from build123d import *

# Parameters (mm, degrees)
PAD_DEPTH       = 100
POCKET_DEPTH    = 35
SKETCH002_W     = 180
SKETCH002_H     = 35
POCKET001_DEPTH = 77
POCKET002_DEPTH = 27


with BuildPart() as part:
    # Sketch001 → Pad (new body)
    with BuildSketch(Plane.XY):
        with BuildLine():
            ThreePointArc((99, 7.5), (80.254858, 52.75481), (35.000067, 71.5))
            Line((35.000067, 71.5), (-35, 71.5))
            ThreePointArc((-35, 71.5), (-80.254834, 52.754834), (-99, 7.5))
            Line((-99, 7.5), (-99, -7.5))
            ThreePointArc((-99, -7.5), (-80.254834, -52.754834), (-35, -71.5))
            Line((-35, -71.5), (35.000001, -71.5))
            ThreePointArc((35.000001, -71.5), (80.254834, -52.754834), (99, -7.5))
            Line((99, 7.5), (99, -7.5))
        make_face()
    extrude(amount=PAD_DEPTH)

    # Sketch → Pocket (cut)
    with BuildSketch(Plane.XY.offset(30)):
        with BuildLine():
            ThreePointArc((89, 7.5), (73.183766, 45.683767), (34.999999, 61.5))
            Line((34.999999, 61.5), (-35, 61.5))
            ThreePointArc((-35, 61.5), (-73.183766, 45.683766), (-89, 7.5))
            Line((-89, 7.5), (-89, -7.5))
            ThreePointArc((-89, -7.5), (-73.183766, -45.683766), (-35, -61.5))
            Line((-35, -61.5), (35, -61.5))
            ThreePointArc((35, -61.5), (73.183766, -45.683766), (89, -7.5))
            Line((89, 7.5), (89, -7.5))
        make_face()
    extrude(amount=POCKET_DEPTH, mode=Mode.SUBTRACT)

    # Sketch002 → Pocket001 (cut)
    with BuildSketch(Plane.XZ.offset(80)):
        with Locations((0, 47.5)):
            Rectangle(SKETCH002_W, SKETCH002_H)
    extrude(amount=-POCKET001_DEPTH, mode=Mode.SUBTRACT)

    # Sketch003 → Pocket002 (cut)
    with BuildSketch(Plane.XY):
        with BuildLine():
            ThreePointArc((96, 7.5), (78.133514, 50.633513), (35.000001, 68.5))
            Line((35.000001, 68.5), (-35, 68.5))
            ThreePointArc((-35, 68.5), (-78.133514, 50.633514), (-96, 7.5))
            Line((-96, 7.5), (-96, -7.5))
            ThreePointArc((-96, -7.5), (-78.133514, -50.633514), (-35, -68.5))
            Line((-35, -68.5), (34.999897, -68.5))
            ThreePointArc((34.999897, -68.5), (78.133477, -50.63355), (96, -7.5))
            Line((96, 7.5), (96, -7.5))
        make_face()
    extrude(amount=POCKET002_DEPTH, mode=Mode.SUBTRACT)


solid = part.part
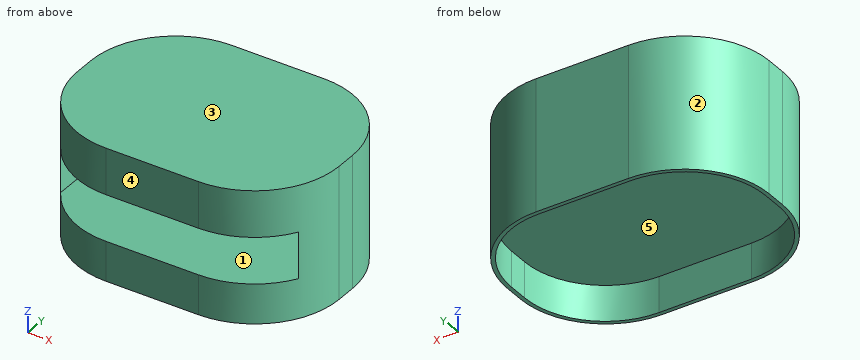
Verification items for the finished model (mm, model axes). Face numbers are marked on the shaded views. A direction names the side the tool comes from. Give positions to 0.01 mm unless a question says otherwise; leave off trailing zeros. Write each loop counter-clockwise with the first axis right and the second up, starting at its lowest first coordinate (ties: lowest second). Pieces come first, ordered by that corner, then holes.
(1) Cross-section at C-C (y = 52). Enter the section's corners in (x, z), plus the area to 3 significant figures.
(2) Access from +Z, -Z, +X, -X, +Y, -Y to the whole of each face (thin tool, end or side, straight path). Record for the marked faces 4 and 5.
(3) Material ranges on line 1 (Z direction, x = 33, y = 61); line 2 (Y direction, x = 32, z = 26); line 3 (Y direction, x = 22, z = 43), recorded low to high.
(4) Gauge pin test, flat ends, axial feed: pin 1 (2 mm diameter, centred on x = -72, z = 63.5, fed in from +Y) (3 decimals); pin 2 (2 mm diameter, centred on y = 31, z = 23, fed in from -X); pin 3 (1.5 mm diameter, centred on x = 30.5, y = -18.5, fed in from -Z); pin 4 (17.5 mm diameter, centred on y = -13.5, z = 49, fed in from -X). Record the tip position at first contact, or that the pin passes through.
(5) Cross-section at D-D (x = -4.5). Enter the section's corners in (y, z), plus the area to 3 significant figures.
(6) Cross-section at A-A (z = 18). Enter the section's corners in (x, y), plus the area to 3 significant figures.
(7) Cross-section at B-B (z = 88). Enter the section's corners in (x, y), plus the area to 3 significant figures.
(8) Mould release check, pull along Z, two halves, no side actions. Record for the marked faces 1, 2 and 3: +Z half, -Z half, draft (parallel to the pull), parting line (faces both ways), or undercut.
Worked out:
1. outline: (-81, 0) - (-76.72, 0) - (-76.72, 27) - (76.72, 27) - (76.72, 0) - (81, 0) - (81, 100) - (-81, 100) - close; hole (-65.59, 30) - (65.59, 30) - (65.59, 65) - (-65.59, 65) - close
1. area: 7,470 mm2
2. face 4: +Z, -Z, +X, -X, -Y
2. face 5: -Z
3. line 1: z = 27 to 30, 65 to 100
3. line 2: y = -71.5 to -68.5, 68.5 to 71.5
3. line 3: y = 61.5 to 71.5
4. pin 1: stops at y = 60.415
4. pin 2: stops at x = -94.91
4. pin 3: stops at z = 27
4. pin 4: stops at x = -99
5. outline: (-71.5, 0) - (-68.5, 0) - (-68.5, 27) - (68.5, 27) - (68.5, 0) - (71.5, 0) - (71.5, 100) - (-71.5, 100) - (-71.5, 65) - (61.5, 65) - (61.5, 30) - (-71.5, 30) - close
5. area: 5,950 mm2
6. outline: (-99, -7.5) arc R64 ccw to (-35, -71.5) - (35, -71.5) arc R64 ccw to (99, -7.5) - (99, 7.5) arc R64 ccw to (35, 71.5) - (-35, 71.5) arc R64 ccw to (-99, 7.5) - close; hole (-96, -7.5) arc R61 ccw to (-35, -68.5) - (35, -68.5) arc R61 ccw to (96, -7.5) - (96, 7.5) arc R61 ccw to (35, 68.5) - (-35, 68.5) arc R61 ccw to (-96, 7.5) - close
6. area: 1,690 mm2
7. outline: (-99, -7.5) arc R64 ccw to (-35, -71.5) - (35, -71.5) arc R64 ccw to (99, -7.5) - (99, 7.5) arc R64 ccw to (35, 71.5) - (-35, 71.5) arc R64 ccw to (-99, 7.5) - close
7. area: 24,800 mm2
8. face 1: undercut
8. face 2: draft
8. face 3: +Z half
